The model under review builds one solid part; all positions refer to its coordinate system, in mm. Coordinates: 2 decimals unless noted, no trailing zeros. Order: outer loops, then holes, each group sorted by start corner. A loop starts at its lowest first (then second) coordinate and runs counter-clockwise, first axis right, second up. Notation, with made-up numbers: (64.5, -30) - (105.5, -30) arc R20 cw to (105.5, -18) - close; hole circle Ø3 at (65, 21.25). An arc over 180 degrees is marked (long way). Answer in a Markdown table with one row per item.
```python
from build123d import *

# Parameters (mm, degrees)
SM_START               = -2
SM_BASE_FLANGE_1_DEPTH = 2
FILLET_1_R             = 5


# Read off the part's stored shape, not the designer's step: 基体-法兰1
with BuildPart() as part:
    # 基体-法兰1 outline → 基体-法兰1 (new body)
    with BuildSketch(Plane.XY.offset(SM_START)):
        with BuildLine():
            Line((-48.022814254, -518.903278649), (-48.022814254, -548.903278649))
            ThreePointArc((-48.022814254, -548.903278649), (0, -551), (48.022814254, -548.903278649))
            Line((48.022814254, -548.903278649), (48.022814254, -518.903278649))
            Line((48.022814254, -518.903278649), (-48.022814254, -518.903278649))
        make_face()
    extrude(amount=SM_BASE_FLANGE_1_DEPTH)

    # 圆角1
    fillet_1_edges = [part.edges().sort_by_distance(p)[0] for p in [
        (-48.022814254, -548.903278649, -1),
        (-48.022814254, -518.903278649, -1),
        (48.022814254, -518.903278649, -1),
        (48.022814254, -548.903278649, -1),
    ]]
    fillet(fillet_1_edges, radius=FILLET_1_R)


solid = part.part
```
Item 1: To check wall thickness, follow line 1 (Y direction, x = -0.5, z = -1.8); line 2 (X direction, y = -523.5, z = -1.55); line 3 (X direction, y = -547.5, z = -1). State the ranges of each line that lie inside material, in increasing order. Write a range as from..to.
Check values:
| item | result |
|---|---|
| line 1 | -551..-518.9 |
| line 2 | -48.01..48.01 |
| line 3 | -46.87..46.87 |
Item 2: Clearance check with flat-ended pins moving along their axes: pin 1 Ø1 at (x, z) = (-34.5, -0.5) entering from -Y; pin 2 Ø5 at (x, y) = (3.5, -542.5) entering from +Z. State where each tip first meets the part, or that it passes through.
Check values:
| item | result |
|---|---|
| pin 1 | y = -549.95 |
| pin 2 | z = 0 |
Item 3: We need section C-C, the plane y = -547. Write out the cut boundary in (x, z), then the cut area to 3 significant figures.
Check values:
| item | result |
|---|---|
| outline | (-47.23, -2) - (47.23, -2) - (47.23, 0) - (-47.23, 0) - close |
| area | 189 mm^2 |
Item 4: We need section B-B, the plane x = -32. Write out the cut boundary in (y, z), then the cut area to 3 significant figures.
Check values:
| item | result |
|---|---|
| outline | (-550.07, -2) - (-518.9, -2) - (-518.9, 0) - (-550.07, 0) - close |
| area | 62.3 mm^2 |
Item 5: We need section A-A, the plane z = -0.3. Write out the cut boundary in (x, y).
Check values:
| item | result |
|---|---|
| outline | (-48.02, -544.3) arc R5 ccw to (-43.42, -549.29) arc R551 ccw to (43.42, -549.29) arc R5 ccw to (48.02, -544.3) - (48.02, -523.9) arc R5 ccw to (43.02, -518.9) - (-43.02, -518.9) arc R5 ccw to (-48.02, -523.9) - close |
